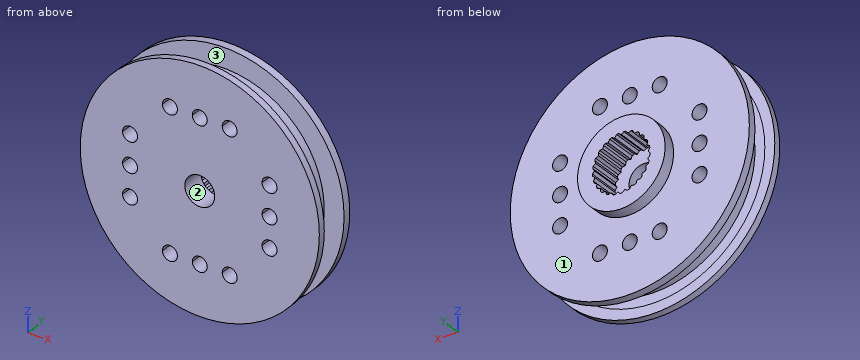
```python
from build123d import *

# Parameters (mm, degrees)
SKETCH2_R               = 6
SKETCH2_R_2             = 1.5
BOSS_EXTRUDE1_DEPTH     = 1.15
SKETCH3_R               = 4.4
BOSS_EXTRUDE2_DEPTH     = 3.2
SKETCH5_R               = 10
SKETCH5_R_2             = 0.75
SKETCH5_R_3             = 1.5
BOSS_EXTRUDE4_DEPTH     = 1.15
ENL_V_START             = -0.6
ESQUISSE4_R             = 10
ESQUISSE4_R_2           = 9
ENL_V_MAT_EXTRU_1_DEPTH = 1
ESQUISSE5_R             = 11.998569968
ESQUISSE5_R_2           = 10
BOSS_EXTRU_1_DEPTH      = 0.55
BOSS_EXTRU_2_START      = -1.6
ESQUISSE5_3_R           = 11.998569968
ESQUISSE5_3_R_2         = 10
BOSS_EXTRU_2_DEPTH      = 0.7
ESQUISSE5_4_R           = 11.998569968
ESQUISSE5_4_R_2         = 10
BOSS_EXTRU_3_DEPTH      = 0.6
ESQUISSE6_R             = 11
ESQUISSE6_R_2           = 9.794741115
BOSS_EXTRU_4_DEPTH      = 1.6
ESQUISSE7_R             = 11.998569968
ESQUISSE7_R_2           = 4.4
BOSS_EXTRU_5_DEPTH      = 2
ENL_V_START_2           = -1
ESQUISSE8_R             = 11.998569968
ESQUISSE8_R_2           = 11
ENL_V_MAT_EXTRU_2_DEPTH = 2.2
ENL_V_START_3           = 10
ESQUISSE9_R             = 0.75
ENL_V_MAT_EXTRU_3_DEPTH = 32.2
ENL_V_START_4           = 1.2
ESQUISSE10_R            = 11.998569968
ESQUISSE10_R_2          = 10.005168165
ENL_V_MAT_EXTRU_4_DEPTH = 2.8


with BuildPart() as part:
    # Sketch2 → Boss-Extrude1 (new body, symmetric)
    with BuildSketch(Plane(origin=(0, 0, 0), x_dir=(1, 0, 0), z_dir=(0, 1, 0))):
        Circle(SKETCH2_R)
        Circle(SKETCH2_R_2, mode=Mode.SUBTRACT)
    extrude(amount=BOSS_EXTRUDE1_DEPTH, both=True)

    # Sketch3 → Boss-Extrude2 (add)
    with BuildSketch(Plane(origin=(0, 1.15, 0), x_dir=(1, 0, 0), z_dir=(0, 1, 0))):
        Circle(SKETCH3_R)
        with BuildLine():
            Line((0.107421435, 2.898009771), (0.338399731, 2.678709694))
            Line((0.338399731, 2.678709694), (0.61665913, 2.83367809))
            ThreePointArc((0.61665913, 2.83367809), (0.721200673, 2.808891167), (0.824752316, 2.780248841))
            Line((0.824752316, 2.780248841), (0.993936292, 2.510396512))
            Line((0.993936292, 2.510396512), (1.301992734, 2.591295993))
            ThreePointArc((1.301992734, 2.591295993), (1.397085655, 2.541289372), (1.490260976, 2.48779465))
            Line((1.490260976, 2.48779465), (1.587020181, 2.184345885))
            Line((1.587020181, 2.184345885), (1.905517346, 2.186093238))
            ThreePointArc((1.905517346, 2.186093238), (1.985186607, 2.11400902), (2.062131058, 2.039023173))
            Line((2.062131058, 2.039023173), (2.080385755, 1.721044772))
            Line((2.080385755, 1.721044772), (2.389311295, 1.643530205))
            ThreePointArc((2.389311295, 1.643530205), (2.448550984, 1.553897705), (2.504429862, 1.46213237))
            Line((2.504429862, 1.46213237), (2.443033042, 1.149604087))
            Line((2.443033042, 1.149604087), (2.722976028, 0.997698125))
            ThreePointArc((2.722976028, 0.997698125), (2.758063897, 0.896149284), (2.789366126, 0.793370413))
            Line((2.789366126, 0.793370413), (2.652175577, 0.505929549))
            Line((2.652175577, 0.505929549), (2.885546163, 0.289177003))
            ThreePointArc((2.885546163, 0.289177003), (2.894277512, 0.182092507), (2.899036259, 0.074758075))
            Line((2.899036259, 0.074758075), (2.694672167, -0.169534403))
            Line((2.694672167, -0.169534403), (2.866806821, -0.437514174))
            ThreePointArc((2.866806821, -0.437514174), (2.848633027, -0.543405812), (2.826549281, -0.648551587))
            Line((2.826549281, -0.648551587), (2.567852594, -0.834345885))
            Line((2.567852594, -0.834345885), (2.667935462, -1.136714727))
            ThreePointArc((2.667935462, -1.136714727), (2.623998452, -1.234759946), (2.576459817, -1.331110368))
            Line((2.576459817, -1.331110368), (2.279685399, -1.446732346))
            Line((2.279685399, -1.446732346), (2.301427906, -1.764491312))
            ThreePointArc((2.301427906, -1.764491312), (2.234488404, -1.84852957), (2.164481907, -1.930030589))
            Line((2.164481907, -1.930030589), (1.848277186, -1.968215294))
            Line((1.848277186, -1.968215294), (1.790313171, -2.281398419))
            ThreePointArc((1.790313171, -2.281398419), (1.704577232, -2.346149284), (1.616501638, -2.40767989))
            Line((1.616501638, -2.40767989), (1.30073492, -2.366028036))
            Line((1.30073492, -2.366028036), (1.166706475, -2.654956874))
            ThreePointArc((1.166706475, -2.654956874), (1.067561203, -2.696351809), (0.966950626, -2.734045809))
            Line((0.966950626, -2.734045809), (0.671462695, -2.615174535))
            Line((0.671462695, -2.615174535), (0.469791321, -2.861694623))
            ThreePointArc((0.469791321, -2.861694623), (0.363466377, -2.877132634), (0.25664255, -2.888621575))
            Line((0.25664255, -2.888621575), (0, -2.7))
            Line((0, -2.7), (-0.25664255, -2.888621575))
            ThreePointArc((-0.25664255, -2.888621575), (-0.363466377, -2.877132634), (-0.469791321, -2.861694623))
            Line((-0.469791321, -2.861694623), (-0.671462695, -2.615174535))
            Line((-0.671462695, -2.615174535), (-0.966950626, -2.734045809))
            ThreePointArc((-0.966950626, -2.734045809), (-1.067561203, -2.696351809), (-1.166706475, -2.654956874))
            Line((-1.166706475, -2.654956874), (-1.30073492, -2.366028036))
            Line((-1.30073492, -2.366028036), (-1.616501638, -2.40767989))
            ThreePointArc((-1.616501638, -2.40767989), (-1.704577232, -2.346149284), (-1.790313171, -2.281398419))
            Line((-1.790313171, -2.281398419), (-1.848277186, -1.968215294))
            Line((-1.848277186, -1.968215294), (-2.164481907, -1.930030589))
            ThreePointArc((-2.164481907, -1.930030589), (-2.234488404, -1.84852957), (-2.301427906, -1.764491312))
            Line((-2.301427906, -1.764491312), (-2.279685399, -1.446732346))
            Line((-2.279685399, -1.446732346), (-2.576459817, -1.331110368))
            ThreePointArc((-2.576459817, -1.331110368), (-2.623998452, -1.234759946), (-2.667935462, -1.136714727))
            Line((-2.667935462, -1.136714727), (-2.567852594, -0.834345885))
            Line((-2.567852594, -0.834345885), (-2.826549281, -0.648551587))
            ThreePointArc((-2.826549281, -0.648551587), (-2.848633027, -0.543405812), (-2.866806821, -0.437514174))
            Line((-2.866806821, -0.437514174), (-2.694672167, -0.169534403))
            Line((-2.694672167, -0.169534403), (-2.899036259, 0.074758075))
            ThreePointArc((-2.899036259, 0.074758075), (-2.894277512, 0.182092507), (-2.885546163, 0.289177003))
            Line((-2.885546163, 0.289177003), (-2.652175577, 0.505929549))
            Line((-2.652175577, 0.505929549), (-2.789366126, 0.793370413))
            ThreePointArc((-2.789366126, 0.793370413), (-2.758063897, 0.896149284), (-2.722976028, 0.997698125))
            Line((-2.722976028, 0.997698125), (-2.443033042, 1.149604087))
            Line((-2.443033042, 1.149604087), (-2.504429862, 1.46213237))
            ThreePointArc((-2.504429862, 1.46213237), (-2.448550984, 1.553897705), (-2.389311295, 1.643530205))
            Line((-2.389311295, 1.643530205), (-2.080385755, 1.721044772))
            Line((-2.080385755, 1.721044772), (-2.062131058, 2.039023173))
            ThreePointArc((-2.062131058, 2.039023173), (-1.985186607, 2.11400902), (-1.905517346, 2.186093238))
            Line((-1.905517346, 2.186093238), (-1.587020181, 2.184345885))
            Line((-1.587020181, 2.184345885), (-1.490260976, 2.48779465))
            ThreePointArc((-1.490260976, 2.48779465), (-1.397085655, 2.541289372), (-1.301992734, 2.591295993))
            Line((-1.301992734, 2.591295993), (-0.993936292, 2.510396512))
            Line((-0.993936292, 2.510396512), (-0.824752316, 2.780248841))
            ThreePointArc((-0.824752316, 2.780248841), (-0.721200673, 2.808891167), (-0.61665913, 2.83367809))
            Line((-0.61665913, 2.83367809), (-0.338399731, 2.678709694))
            Line((-0.338399731, 2.678709694), (-0.107421435, 2.898009771))
            ThreePointArc((-0.107421435, 2.898009771), (0, 2.9), (0.107421435, 2.898009771))
        make_face(mode=Mode.SUBTRACT)
    extrude(amount=BOSS_EXTRUDE2_DEPTH)

    # Sketch5 → Boss-Extrude4 (add, symmetric)
    with BuildSketch(Plane(origin=(0, 0, 0), x_dir=(1, 0, 0), z_dir=(0, 1, 0))):
        Circle(SKETCH5_R)
        with Locations((0, 7)):
            Circle(SKETCH5_R_2, mode=Mode.SUBTRACT)
        with Locations((-3, 7)):
            Circle(SKETCH5_R_2, mode=Mode.SUBTRACT)
        with Locations((3, 7)):
            Circle(SKETCH5_R_2, mode=Mode.SUBTRACT)
        with Locations((7, 3)):
            Circle(SKETCH5_R_2, mode=Mode.SUBTRACT)
        with Locations((7, 0)):
            Circle(SKETCH5_R_2, mode=Mode.SUBTRACT)
        with Locations((7, -3)):
            Circle(SKETCH5_R_2, mode=Mode.SUBTRACT)
        with Locations((3, -7)):
            Circle(SKETCH5_R_2, mode=Mode.SUBTRACT)
        with Locations((0, -7)):
            Circle(SKETCH5_R_2, mode=Mode.SUBTRACT)
        with Locations((-3, -7)):
            Circle(SKETCH5_R_2, mode=Mode.SUBTRACT)
        with Locations((-7, -3)):
            Circle(SKETCH5_R_2, mode=Mode.SUBTRACT)
        with Locations((-7, 0)):
            Circle(SKETCH5_R_2, mode=Mode.SUBTRACT)
        with Locations((-7, 3)):
            Circle(SKETCH5_R_2, mode=Mode.SUBTRACT)
        Circle(SKETCH5_R_3, mode=Mode.SUBTRACT)
    extrude(amount=BOSS_EXTRUDE4_DEPTH, both=True)

    # Esquisse4 → Enl_v. mat.-Extru.1 (cut)
    with BuildSketch(Plane(origin=(0, 1.15, 0), x_dir=(1, 0, 0), z_dir=(0, 1, 0)).offset(ENL_V_START)):
        Circle(ESQUISSE4_R)
        Circle(ESQUISSE4_R_2, mode=Mode.SUBTRACT)
    extrude(amount=-ENL_V_MAT_EXTRU_1_DEPTH, mode=Mode.SUBTRACT)

    # Esquisse5 → Boss.-Extru.1 (add)
    with BuildSketch(Plane(origin=(0, 1.15, 0), x_dir=(1, 0, 0), z_dir=(0, 1, 0))):
        Circle(ESQUISSE5_R)
        Circle(ESQUISSE5_R_2, mode=Mode.SUBTRACT)
    extrude(amount=-BOSS_EXTRU_1_DEPTH)

    # Esquisse5_3 → Boss.-Extru.2 (add)
    with BuildSketch(Plane(origin=(0, 1.15, 0), x_dir=(1, 0, 0), z_dir=(0, 1, 0)).offset(BOSS_EXTRU_2_START)):
        Circle(ESQUISSE5_3_R)
        Circle(ESQUISSE5_3_R_2, mode=Mode.SUBTRACT)
    extrude(amount=-BOSS_EXTRU_2_DEPTH)

    # Esquisse5_4 → Boss.-Extru.3 (add)
    with BuildSketch(Plane(origin=(0, 1.15, 0), x_dir=(1, 0, 0), z_dir=(0, 1, 0))):
        Circle(ESQUISSE5_4_R)
        Circle(ESQUISSE5_4_R_2, mode=Mode.SUBTRACT)
    extrude(amount=-BOSS_EXTRU_3_DEPTH)

    # Esquisse6 → Boss.-Extru.4 (add)
    with BuildSketch(Plane(origin=(0, 1.15, 0), x_dir=(1, 0, 0), z_dir=(0, 1, 0))):
        Circle(ESQUISSE6_R)
        Circle(ESQUISSE6_R_2, mode=Mode.SUBTRACT)
    extrude(amount=-BOSS_EXTRU_4_DEPTH)

    # Esquisse7 → Boss.-Extru.5 (add)
    with BuildSketch(Plane(origin=(0, 1.15, 0), x_dir=(1, 0, 0), z_dir=(0, 1, 0))):
        Circle(ESQUISSE7_R)
        Circle(ESQUISSE7_R_2, mode=Mode.SUBTRACT)
    extrude(amount=BOSS_EXTRU_5_DEPTH)

    # Esquisse8 → Enl_v. mat.-Extru.2 (cut)
    with BuildSketch(Plane(origin=(0, 1.15, 0), x_dir=(1, 0, 0), z_dir=(0, 1, 0)).offset(ENL_V_START_2)):
        Circle(ESQUISSE8_R)
        Circle(ESQUISSE8_R_2, mode=Mode.SUBTRACT)
    extrude(amount=ENL_V_MAT_EXTRU_2_DEPTH, mode=Mode.SUBTRACT)

    # Esquisse9 → Enl_v. mat.-Extru.3 (cut)
    with BuildSketch(Plane(origin=(0, -1.15, 0), x_dir=(-1, 0, 0), z_dir=(0, -1, 0)).offset(ENL_V_START_3)):
        with Locations((3, 7)):
            Circle(ESQUISSE9_R)
        with Locations((7, 3)):
            Circle(ESQUISSE9_R)
        with Locations((7, 0)):
            Circle(ESQUISSE9_R)
        with Locations((7, -3)):
            Circle(ESQUISSE9_R)
        with Locations((3, -7)):
            Circle(ESQUISSE9_R)
        with Locations((0, -7)):
            Circle(ESQUISSE9_R)
        with Locations((-3, -7)):
            Circle(ESQUISSE9_R)
        with Locations((-7, -3)):
            Circle(ESQUISSE9_R)
        with Locations((-7, 0)):
            Circle(ESQUISSE9_R)
        with Locations((-7, 3)):
            Circle(ESQUISSE9_R)
        with Locations((-3, 7)):
            Circle(ESQUISSE9_R)
        with Locations((0, 7)):
            Circle(ESQUISSE9_R)
    extrude(amount=-ENL_V_MAT_EXTRU_3_DEPTH, mode=Mode.SUBTRACT)

    # Esquisse10 → Enl_v. mat.-Extru.4 (cut)
    with BuildSketch(Plane(origin=(0, 1.15, 0), x_dir=(1, 0, 0), z_dir=(0, 1, 0)).offset(ENL_V_START_4)):
        Circle(ESQUISSE10_R)
        Circle(ESQUISSE10_R_2, mode=Mode.SUBTRACT)
    extrude(amount=-ENL_V_MAT_EXTRU_4_DEPTH, mode=Mode.SUBTRACT)


solid = part.part
```
Model file for the job. Use its own axes, mm. Face numbers are marked on the shaded views. Give positions to 0.01 mm unless a question says otherwise; leave off trailing zeros. Write each loop counter-clockwise with the first axis right and the second up, starting at its lowest first coordinate (ties: lowest second). Pieces come first, ordered by that corner, then holes. Notation, with made-up numbers: (36, 43) - (87, 43) arc R7 cw to (87, 48) - close; hole circle Ø6 at (32, -11). An arc over 180 degrees is marked (long way). One line per question, with ' | ' between items. Start each with the question number.
(1) Slice it at A-A on x = -7. Give the number of separate pieces and of enclosed holes in the cut face, plus the area to 3 significant figures.
(2) Wall check: line 1 along Z through (x, y) = (0, -0.4); line 2 along Z through (x, y) = (3, 2.1). Give the ranges that are in metal, low to high. Write a range as from..to.
(3) Slice it at D-D on x = 5.75. Write the cut outline in (y, z), plus the area to 3 significant figures.
(4) Pin check, flat tips, straight feed: P1, Ø1, axis at x = -2.5, y = 2, coming from the +Z side; P2, Ø1, axis at y = 2.5, z = -1, coming from the -X side; P3, Ø1.2, axis at x = 7, z = -3, coming from the +Y side; P4, Ø1.7, axis at x = 0, z = -7, coming from the +Y side. Stop position of each tip, or through.
(5) Two-plate mould, pull along Y, no slides. Class the marked faces 1, 2 and 3: +Y half, -Y half, draft (parallel to the pull), parting line (faces both ways), or undercut.
Results below:
1) separate pieces: 4 | enclosed holes: 2 | area: 47.5 mm^2
2) line 1: -10.01..-9.79, -9..-7.75, -6.25..-1.5, 1.5..6.25, 7.75..9, 9.79..10.01 | line 2: -9.54..-7.75, -6.25..6.25, 7.75..9.54
3) outline: (-1.15, -10.53) - (-0.45, -10.53) - (-0.45, -8.19) - (2.35, -8.19) - (2.35, -10.53) - (3.15, -10.53) - (3.15, 10.53) - (2.35, 10.53) - (2.35, 8.19) - (-0.45, 8.19) - (-0.45, 10.53) - (-1.15, 10.53) - close; hole (-0.45, -7.93) - (0.55, -7.93) - (0.55, -6.92) - (-0.45, -6.92) - close; hole (-0.45, 6.92) - (0.55, 6.92) - (0.55, 7.93) - (-0.45, 7.93) - close | area: 75.4 mm^2
4) P1: z = 11.81 | P2: x = -11.99 | P3: through | P4: y = 3.15
5) face 1: +Y half | face 2: draft | face 3: undercut
